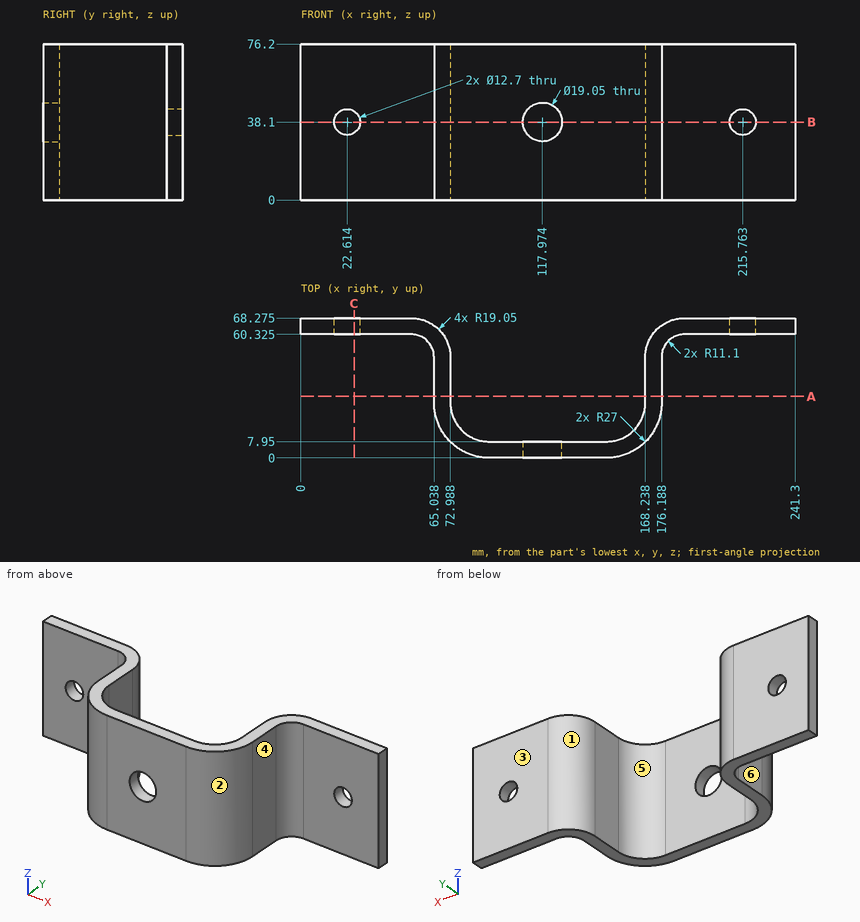
Design review of the part shown in the three views and the two pictorial views. Dimensions are in mm from the part's minimum x, y and z. A direction names the side the tool comes from. Round coordinates to 2 decimals unless told otherwise and drop trailing zeros. Order: outer loops, then holes, each group sorted by start corner. A loop starts at its lowest first (then second) coordinate and runs counter-clockwise, first axis right, second up. Notation, with made-up numbers: (38.5, 7) - (49.5, 7) arc R15 ccw to (49.5, 16) - close; hole circle Ø11 at (34, 63.25). An arc over 180 degrees is marked (long way). Answer in a Markdown table with one row per item.
(1) Take a section at B-B on z = 38.1. Count the separate pieces of the cut face and the enclosed holes in it, plus the area to 3 significant figures.
Result set:
| item | result |
|---|---|
| separate pieces | 4 |
| enclosed holes | 0 |
| area | 2,260 mm2 |
(2) For line 1 (X direction, y = 63, z = 38) (1 decimal); line 2 (X direction, y = 26, z = 41.5); line 3 (X direction, y = 22, z = 53) (1 decimal), list the stretches that pass through material, from the lowest coordinate up. Write a range as from..to.
Result set:
| item | result |
|---|---|
| line 1 | x = 0..16.3, 29..67.1, 174.1..209.4, 222.1..241.3 |
| line 2 | x = 65.06..73.01, 168.21..176.17 |
| line 3 | x = 65.5..73.7, 167.6..175.7 |
(3) Take a section at A-A on y = 30. Write out the cut boundary in (x, z).
Result set:
| item | result |
|---|---|
| outline | (65.04, 0) - (72.99, 0) - (72.99, 76.2) - (65.04, 76.2) - close; (168.24, 0) - (176.19, 0) - (176.19, 76.2) - (168.24, 76.2) - close |
(4) Clearance check with flat-ended pins moving along their axes: P1, Ø1.5, axis at y = 35, z = 51, coming from the -X side; P2, Ø6.5, axis at y = 37, z = 25, coming from the +X side; P3, Ø10, axis at x = 215.76, z = 38.1, coming from the +Y side; P4, Ø6, axis at x = 61.5, z = 56.5, coming from the +Y side. State where each tip first meets the part, or that it passes through.
Result set:
| item | result |
|---|---|
| P1 | stops at x = 65.04 |
| P2 | stops at x = 176.19 |
| P3 | passes through |
| P4 | stops at y = 67.72 |
(5) Machinability: for the marked faces 4, 5 and 6, which of the approach directions +Z, -Z, +X, -X, +Y, -Y give a long, thin tool a straight path to every point of the face, cutting with its end or side? Answer none if there is none.
Result set:
| item | result |
|---|---|
| face 4 | +Z, -Z, +X, -Y |
| face 5 | +Z, -Z, +Y |
| face 6 | +Z, -Z, -X, -Y |
(6) Take a section at C-C on x = 26. Write out the cut boundary in (y, z) (1 decimal).
Result set:
| item | result |
|---|---|
| outline | (60.3, 0) - (68.3, 0) - (68.3, 32.7) - (60.3, 32.7) - close; (60.3, 43.5) - (68.3, 43.5) - (68.3, 76.2) - (60.3, 76.2) - close |
(7) Mouldability with a two-part tool opening along X and no side actions: class the marked faces 1, 2 and 3 as released by +X, released by -X, zero draft, split by the parting line, or undercut.
Result set:
| item | result |
|---|---|
| face 1 | undercut |
| face 2 | released by +X |
| face 3 | zero draft |
